Source: CAD feature listing. Evaluate the final solid. Frame: model axes, mm. A direction names the side the tool comes from. Give positions to 0.01 mm unless a question says otherwise; leave off trailing zeros. Order: outer loops, then holes, each group sorted by start corner. A loop starts at its lowest first (then second) coordinate and runs counter-clockwise, first axis right, second up. Notation, with made-up numbers: M 86.25,76.25 L 90.25,76.25 A20 cw 90.25,108.25 Z; hole C 45.5,28.25 d10. An arc over 180 degrees is marked long. Use CSV: the item, a comma, the result in double quotes. Start each with the question number.
Item 1: Section query D-D on y = 4.75. Return loops of the section in (x, z), and give its area (3 significant figures).
Item 2: Pull-direction query (X, two-part tool) for faces 3 (the face through (0, 10, 0)), 4 (the face through (7.81, 11.53, 1.73)), 5 (the face through (6, 9, -2)); classes: +X half, -X half, draft (parallel to the pull), parting line (faces both ways), or undercut.
Item 3: Section query C-C on y = 9.75. Return loops of the section in (x, z), and give its area (3 significant figures).
Item 4: Access query for faces 1 (the face through (-4.5, 4.9, -3.5)), 2 (the face through (0, 14, 0)). Directions: +Z, -Z, +X, -X, +Y, -Y. A direction counts if a zero-diameter tool reaches every point of the face in a straight line with its end or side. Return the directions, or none.
Item 5: Section query B-B on z = 0. Return loops of the section in (x, y), and give its area (3 significant figures).
Item 6: Section query A-A on x = 0. Return loops of the section in (y, z), and give its area (3 significant figures).
Item 7: First-contact query: pin 1 (1 mm diameter, centred on y = 10, z = 3.5, fed in from -X); pin 2 (1.5 mm diameter, centred on x = -3.5, y = 9, fed in from -Z); pin 3 (5 mm diameter, centred on x = -2.5, y = 3.5, fed in from +Z). Flat tips, straight axial feed; report the tip coordinate or a pass-through.
Item 8: Ray query, probe 1 along Y at (x, z) = (4.25, 4.5); probe 2 along Y at (x, z) = (-0.5, 0.5); probe 3 along X at (y, z) = (6.5, -1.75). Return the intervals inside material, ascending. Write a range as from..to.
Autodesk Inventor part; units mm, degrees
ref_plane "YZ Plane" through (0, 0, 0) normal (1, 0, 0) x (0, 1, 0)
ref_plane "XZ Plane" through (0, 0, 0) normal (0, 1, 0) x (-1, 0, 0)
ref_plane "XY Plane" through (0, 0, 0) normal (0, 0, 1) x (1, 0, 0)
sketch "Szkic2" plane through (0, 0, 0) normal (1, 0, 0) x (0, 1, 0)
  line L0 (0, 0) -> (0, -6)
  line L1 (0, -6) -> (9, -6)
  line L2 (9, -6) -> (9, -8)
  line L3 (9, -8) -> (14, -8)
  line L4 (14, -8) -> (14, 0)
  line L5 (14, 0) -> (0, 0)
  dimension "d6" = 6
  dimension "d7" = 9
  dimension "d8" = 2
  dimension "d9" = 5
revolve "Obrót1" add sketch "Szkic2" angle 360 about axis through (0, 14, 0) along (0, -1, 0)
sketch "Szkic3" plane through (0, 0, 0) normal (0, -1, 0) x (1, 0, 0)
  circle A0 centre (0, 0) radius 6
  circle A1 centre (0, 0) radius 5.7
  dimension "d11" = 11.4
extrude "Wyciągnięcie proste1" cut sketch "Szkic3" against normal blind 10 contours A1
fillet "Zaokrąglenie1" radius 0.5 2 edges at (0, 9, 8) (0, 14, 8)
properties material "Kauczuk"
Verdict:
1,outline,"C 0,0 d12; hole C 0,0 d11.4"
1,area,"11.0 mm2"
2,face 3,"undercut"
2,face 4,"parting line"
2,face 5,"draft"
3,outline,"C 0,0 d16; hole C 0,0 d11.4"
3,area,"99.0 mm2"
4,face 1,"-Y"
4,face 2,"+Z, -Z, +X, -X, +Y"
5,outline,"M -8,9.5 A0.5 ccw -7.5,9 L -6,9 L -6,0 L -5.7,0 L -5.7,10 L 5.7,10 L 5.7,0 L 6,0 L 6,9 L 7.5,9 A0.5 ccw 8,9.5 L 8,13.5 A0.5 ccw 7.5,14 L -7.5,14 A0.5 ccw -8,13.5 Z"
5,area,"73.8 mm2"
6,outline,"M 0,-6 L 9,-6 L 9,-7.5 A0.5 ccw 9.5,-8 L 13.5,-8 A0.5 ccw 14,-7.5 L 14,7.5 A0.5 ccw 13.5,8 L 9.5,8 A0.5 ccw 9,7.5 L 9,6 L 0,6 L 0,5.7 L 10,5.7 L 10,-5.7 L 0,-5.7 Z"
6,area,"73.8 mm2"
7,pin 1,"x = -7.42"
7,pin 2,"z = -7.46"
7,pin 3,"z = 6"
8,probe 1,"9..14"
8,probe 2,"10..14"
8,probe 3,"-5.74..-5.42, 5.42..5.74"
